Build history of the part. All positions in model axes, mm. Round coordinates to 2 decimals unless told otherwise and drop trailing zeros. Order: outer loops, then holes, each group sorted by start corner. A loop starts at its lowest first (then second) coordinate and runs counter-clockwise, first axis right, second up. Notation, with made-up numbers: (87.25, 58) -> (132.25, 58) arc R16 ccw to (132.25, 70) -> close; hole circle Ø10 at (-10.5, 60.25). An arc over 180 degrees is marked (long way). Write item = value, one per line.
from build123d import *

# Parameters (mm, degrees)
SKETCH1_W                    = 25.4
SKETCH1_H                    = 25.4
SKETCH1_W_2                  = 15.875
SKETCH1_H_2                  = 279.4
BOSS_EXTRUDE1_DEPTH          = 3.175
F_25_0_1495_DIAMETER_HOLE2_D = 3.7973
SKETCH4_W                    = 304.8
SKETCH4_H                    = 3.175
BOSS_EXTRUDE2_DEPTH          = 17.78
SKETCH5_R                    = 0.127
CUT_EXTRUDE1_DEPTH           = 4.175
F_25_0_1495_DIAMETER_HOLE1_D = 3.7973


with BuildPart() as part:
    # Sketch1 → Boss-Extrude1 (new body)
    with BuildSketch(Plane(origin=(0, 0, 0), x_dir=(1, 0, 0), z_dir=(0, 1, 0))):
        with Locations((12.7, 292.1)):
            Rectangle(SKETCH1_W, SKETCH1_H)
        with Locations((33.3375, 292.1)):
            Rectangle(SKETCH1_W_2, SKETCH1_H)
        with Locations((12.7, 139.7)):
            Rectangle(SKETCH1_W, SKETCH1_H_2)
    extrude(amount=BOSS_EXTRUDE1_DEPTH)

    # #25 (0.1495) Diameter Hole2 (through all)
    with Locations(Plane(origin=(0, 3.175, 0), x_dir=(1, 0, 0), z_dir=(0, 1, 0))):
        with Locations((10.16, 16.51), (10.16, 73.308346978), (10.16, 140.97), (33.02, 298.45)):
            Hole(F_25_0_1495_DIAMETER_HOLE2_D / 2)

    # Sketch4 → Boss-Extrude2 (add)
    with BuildSketch(Plane.ZY):
        with Locations((-152.4, 1.5875)):
            Rectangle(SKETCH4_W, SKETCH4_H)
    extrude(amount=BOSS_EXTRUDE2_DEPTH)

    # Sketch5 → Cut-Extrude1 (cut, through all)
    with BuildSketch(Plane(origin=(0, 3.175, 0), x_dir=(1, 0, 0), z_dir=(0, 1, 0))):
        with Locations((-6.223, 42.799)):
            Circle(SKETCH5_R)
        with Locations((-6.223, 22.479)):
            Circle(SKETCH5_R)
        with Locations((-6.223, 63.119)):
            Circle(SKETCH5_R)
        with Locations((-6.223, 83.439)):
            Circle(SKETCH5_R)
        with Locations((-6.223, 103.759)):
            Circle(SKETCH5_R)
        with Locations((-6.223, 124.079)):
            Circle(SKETCH5_R)
        with Locations((-6.223, 144.399)):
            Circle(SKETCH5_R)
    extrude(amount=-CUT_EXTRUDE1_DEPTH, mode=Mode.SUBTRACT)

    # #25 (0.1495) Diameter Hole1 (through all)
    with Locations(Plane(origin=(0, 3.175, 0), x_dir=(1, 0, 0), z_dir=(0, 1, 0))):
        with Locations((-6.223, 42.799), (-6.223, 63.119), (-6.223, 83.439), (-6.223, 103.759), (-6.223, 124.079), (-6.223, 144.399), (-6.223, 22.479)):
            Hole(F_25_0_1495_DIAMETER_HOLE1_D / 2)


solid = part.part
Q1. Cut at A-A, the plane y = 2.55. Give the number of separate pieces and of enclosed holes in the cut face, and give its area (3 significant figures).
Check values:
separate_pieces = 1
enclosed_holes = 11
area = 13,400 mm²
Q2. Flat gauge pins, fed straight in: pin 1 (1 mm diameter, centred on y = 1.5, z = -117, fed in from +X); pin 2 (1 mm diameter, centred on x = 34, y = 1, fed in from +Z). Where does each tip first touch, or does it go through?
Check values:
pin_1 = 25.4
pin_2 = -279.4
Q3. Probe probe 1 along X at (y, z) = (1.55, -83); probe 2 along X at (y, z) = (2.55, -298.45) (3 decimals); probe 3 along Z at (x, y) = (25.5, 1.65). List the from-to ranges inside material, lowest first.
Check values:
probe_1 = -17.78 to -8.07, -4.38 to 25.4
probe_2 = -17.78 to 31.121, 34.919 to 41.275
probe_3 = -304.8 to -279.4
Q4. Cut at B-B, the plane z = -171.5. List the corners of the cut face in (x, y) (3 decimals).
Check values:
outline = (-17.78, 0) -> (25.4, 0) -> (25.4, 3.175) -> (-17.78, 3.175) -> close
